Read the model definition and answer for the solid it produces. Units are mm, in the model's axes. A direction names the side the tool comes from. Coordinates: 2 decimals unless noted, no trailing zeros. Loops run counter-clockwise (first coordinate to the right, second up) from the corner with the lowest first, then second, coordinate; pieces in that order, holes last. Notation, with made-up numbers: (22.25, 5) -> (37.25, 5) arc R25 ccw to (37.25, 33) -> close; hole circle Ø9 at (-16.5, 63.5). An arc over 180 degrees is marked (long way). Answer as a JSON object with one key per item and string values. Group by question number.
Q1. The part is cut by section A-A on y = -30. Write down the section's boundary in (x, z), and give its area (3 significant figures).
Q2. For faces 5 (the cylindrical face through (84, 22, 25)), 6 (the flat face through (83, 0, 12)), 7 (the cylindrical face through (13.93, -11.5, 1.48)), 8 (the flat face through (3, 11, 27)), determine the directions among +Z, -Z, +X, -X, +Y, -Y from which every point of the face is accessible in a straight line to the end or side of a thin tool.
Q3. The part is cut by section C-C on y = 11.5. State how many separate pieces and enclosed holes the cut face has, and give its area (3 significant figures).
Q4. The part is cut by section D-D on x = 51. Write down the section's boundary in (y, z).
Q5. The part is cut by section B-B on z = 25. Write down the section's boundary in (x, y), and give its area (3 significant figures).
Q6. Determine the mould class of faces 1 (the cylindrical face through (83.521, 10.979, 17.466)), 2 (the cylindrical face through (71, -11.43, 1.48)), 3 (the cylindrical face through (1.521, 10.979, 17.466)), 4 (the flat face through (82, 14, 17)) for opening direction Y: released by +Y, released by -Y, zero draft, split by the parting line, or undercut.
Q7. Straight lines are drawn through the part: line 1 along X through (y, z) = (16.5, 5.5); line 2 along Y through (x, z) = (83, 13); line 3 along X through (y, z) = (18, 45.5). For each, find the intervals that lie inside material, in ascending order. Write a range as [from, to].
Q8. This flat-tipped pin is pushed along its axis until it touches: P1, Ø1.5, axis at x = 1, z = 16.5, coming from the -Y side. Where does it stop, or does it pass through?
from build123d import *

# Parameters (mm, degrees)
F0_W     = 85
F0_H     = 23
F1_DEPTH = 3
F2_W     = 3
F2_H     = 23
F3_DEPTH = 24
F4_W     = 3
F4_H     = 23
F5_DEPTH = 25
F6_R     = 4
F6_R_2   = 2
F7_DEPTH = 250
F8_R     = 5


with BuildPart() as f1:
    # F0 (on Top) → F1 (new body)
    with BuildSketch(Plane.XY):
        with Locations((42.5, 11.5)):
            Rectangle(F0_W, F0_H)
        with BuildLine():
            Line((85, 0), (0, 0))
            Line((0, 0), (0, -10))
            Line((0, -10), (0, -65))
            ThreePointArc((0, -65), (1.464466, -68.535534), (5, -70))
            Line((5, -70), (7.5, -70))
            ThreePointArc((7.5, -70), (11.035534, -68.535534), (12.5, -65))
            Line((12.5, -65), (12.5, -15))
            ThreePointArc((12.5, -15), (13.964466, -11.464466), (17.5, -10))
            Line((17.5, -10), (67.5, -10))
            ThreePointArc((67.5, -10), (71.035534, -11.464466), (72.5, -15))
            Line((72.5, -15), (72.5, -65))
            ThreePointArc((72.5, -65), (73.964466, -68.535534), (77.5, -70))
            Line((77.5, -70), (80, -70))
            ThreePointArc((80, -70), (83.535534, -68.535534), (85, -65))
            Line((85, -65), (85, -10))
            Line((85, -10), (85, 0))
        make_face()
    extrude(amount=F1_DEPTH)

    # F2 (on face) → F3 (join)
    with BuildSketch(Plane.XY.offset(3)):
        with Locations((1.5, 11.5)):
            Rectangle(F2_W, F2_H)
        with Locations((83.5, 11.5)):
            Rectangle(F2_W, F2_H)
    extrude(amount=F3_DEPTH)

    # F4 (on face) → F5 (join)
    with BuildSketch(Plane.XY.offset(27)):
        with Locations((1.5, 11.5)):
            Rectangle(F4_W, F4_H)
    extrude(amount=F5_DEPTH)

    # F6 (on face) → F7 (cut)
    with BuildSketch(Plane.YZ.offset(85)):
        with Locations((11.5, 13.5)):
            Circle(F6_R)
        with Locations((5.843146, 19.156854)):
            Circle(F6_R_2)
        with Locations((11.5, 21.5)):
            Circle(F6_R_2)
        with Locations((17.156854, 19.156854)):
            Circle(F6_R_2)
        with Locations((19.5, 13.5)):
            Circle(F6_R_2)
        with Locations((17.156854, 7.843146)):
            Circle(F6_R_2)
        with Locations((11.5, 5.5)):
            Circle(F6_R_2)
        with Locations((5.843146, 7.843146)):
            Circle(F6_R_2)
        with Locations((3.5, 13.5)):
            Circle(F6_R_2)
    extrude(amount=-F7_DEPTH, mode=Mode.SUBTRACT)

    # F8
    f8_edges = [f1.edges().sort_by_distance(p)[0] for p in [
        (1.5, 23, 52),
        (1.5, 0, 52),
        (83.5, 23, 27),
        (83.5, 0, 27),
    ]]
    fillet(f8_edges, radius=F8_R)


solid = f1.part
Final values:
{
 "1": {"outline": "(0, 0) -> (12.5, 0) -> (12.5, 3) -> (0, 3) -> close; (72.5, 0) -> (85, 0) -> (85, 3) -> (72.5, 3) -> close", "area": "75.0 mm2"},
 "2": {"face 5": "+Z, +X, +Y", "face 6": "+Z, +X, -X, -Y", "face 7": "+Z, -Z, -Y", "face 8": "+Z, +Y, -Y"},
 "3": {"separate pieces": "7", "enclosed holes": "0", "area": "378 mm2"},
 "4": {"outline": "(-10, 0) -> (23, 0) -> (23, 3) -> (-10, 3) -> close"},
 "5": {"outline": "(0, 0) -> (3, 0) -> (3, 23) -> (0, 23) -> close; (82, 1) -> (85, 1) -> (85, 22) -> (82, 22) -> close", "area": "132 mm2"},
 "6": {"face 1": "undercut", "face 2": "released by -Y", "face 3": "undercut", "face 4": "zero draft"},
 "7": {"line 1": "x = [0, 3], [82, 85]", "line 2": "y = [0, 1.56], [5.44, 7.53], [15.47, 17.56], [21.44, 23]", "line 3": "x = [0, 3]"},
 "8": {"P1": "stops at y = 0"}
}
